Build history of the part. All positions in model axes, mm. Round coordinates to 2 decimals unless told otherwise and drop trailing zeros. Write each loop counter-clockwise with the first axis right and the second up, starting at its lowest first coordinate (ties: lowest second). Pieces come first, ordered by that corner, then holes. Notation, with made-up numbers: (84, 80) -> (128, 80) arc R15 cw to (128, 89) -> close; hole circle Ø1 at (57.5, 57). An arc over 180 degrees is marked (long way). Return JSON: item names as keys, results as strings.
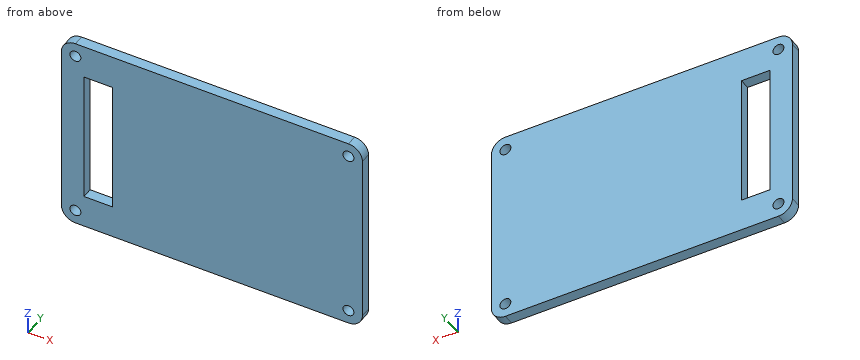
from build123d import *

# Parameters (mm, degrees)
SKETCH2_R           = 1.63195
BOSS_EXTRUDE3_DEPTH = 3.175
SKETCH3_W           = 8.5
SKETCH3_H           = 40
CUT_EXTRUDE1_DEPTH  = 55.176384385


with BuildPart() as part:
    # Sketch2 → Boss-Extrude3 (new body)
    with BuildSketch(Plane(origin=(0, 0, 0), x_dir=(1, 0, 0), z_dir=(0, 1, 0))):
        with BuildLine():
            Line((-45, 25.825), (-45, -25.825))
            ThreePointArc((-45, -25.825), (-43.777170811, -28.777170811), (-40.825, -30))
            Line((-40.825, -30), (40.825, -30))
            ThreePointArc((40.825, -30), (43.777170811, -28.777170811), (45, -25.825))
            Line((45, -25.825), (45, 25.825))
            ThreePointArc((45, 25.825), (43.777170811, 28.777170811), (40.825, 30))
            Line((40.825, 30), (-40.825, 30))
            ThreePointArc((-40.825, 30), (-43.777170811, 28.777170811), (-45, 25.825))
        make_face()
        with Locations(Location((40.825, 25.825, 0), (0, 0, 270))):
            Circle(SKETCH2_R, mode=Mode.SUBTRACT)
        with Locations(Location((40.825, -25.825, 0), (0, 0, 270))):
            Circle(SKETCH2_R, mode=Mode.SUBTRACT)
        with Locations(Location((-40.825, 25.825, 0), (0, 0, 270))):
            Circle(SKETCH2_R, mode=Mode.SUBTRACT)
        with Locations(Location((-40.825, -25.825, 0), (0, 0, 270))):
            Circle(SKETCH2_R, mode=Mode.SUBTRACT)
    extrude(amount=BOSS_EXTRUDE3_DEPTH)

    # Sketch3 → Cut-Extrude1 (cut, through all)
    with BuildSketch(Plane(origin=(0, 3.175, 0), x_dir=(1, 0, 0), z_dir=(0, 1, 0))):
        with Locations((-34.015313808, 0.1)):
            Rectangle(SKETCH3_W, SKETCH3_H)
    extrude(amount=-CUT_EXTRUDE1_DEPTH, mode=Mode.SUBTRACT)


solid = part.part
Q1. Saw through at A-A on z = -5. List the corners of the cut face in (x, y) (3 decimals).
Verdict:
{"outline": "(-45, 0) -> (-38.265, 0) -> (-38.265, 3.175) -> (-45, 3.175) -> close; (-29.765, 0) -> (45, 0) -> (45, 3.175) -> (-29.765, 3.175) -> close"}
Q2. Saw through at B-B on y = 2. List the corners of the cut face in (x, z) (3 decimals), then the cut area to 3 significant figures.
Verdict:
{"outline": "(-45, -25.825) arc R4.175 ccw to (-40.825, -30) -> (40.825, -30) arc R4.175 ccw to (45, -25.825) -> (45, 25.825) arc R4.175 ccw to (40.825, 30) -> (-40.825, 30) arc R4.175 ccw to (-45, 25.825) -> close; hole circle Ø3.264 at (-40.825, -25.825); hole circle Ø3.264 at (-40.825, 25.825); hole (-38.265, -20.1) -> (-29.765, -20.1) -> (-29.765, 19.9) -> (-38.265, 19.9) -> close; hole circle Ø3.264 at (40.825, -25.825); hole circle Ø3.264 at (40.825, 25.825)", "area": "5,010 mm²"}
Q3. Pin check, flat tip, straight feed: pin 1 Ø5 at (x, z) = (-40.825, -25.825) entering from +Y (3 decimals). Stop position of the tip, or through.
Verdict:
{"pin 1": "stops at y = 3.175"}
Q4. Wall check: L1, parallel to X at y = 0.8, z = -11; L2, parallel to Z at x = -36, y = 2.5. Give the ranges that are in metal, low to high.
Verdict:
{"L1": "x = -45 to -38.27, -29.77 to 45", "L2": "z = -30 to -20.1, 19.9 to 30"}
